```python
from build123d import *

# Parameters (mm, degrees)
F1_DEPTH = 76.2
F3_DEPTH = 38.101


with BuildPart() as f1:
    # F0 (on Front) → F1 (new body)
    with BuildSketch(Plane.XZ):
        Polygon((0, 101.6), (0, 0), (152.4, 0), (152.4, 38.1), (38.1, 38.1), (38.1, 101.6), align=None)
    extrude(amount=F1_DEPTH)

    # F2 (on face) → F3 (cut, through all)
    with BuildSketch(Plane.YZ.offset(38.1)):
        Polygon((-76.2, 69.85), (-38.1, 101.6), (-76.2, 101.6), align=None)
    extrude(amount=-F3_DEPTH, mode=Mode.SUBTRACT)


solid = f1.part
```
Here's how the part is built. I have some questions about the finished solid (model axes, mm). A direction names the side the tool comes from. Coordinates: 2 decimals unless noted, no trailing zeros. Write each loop counter-clockwise with the first axis right and the second up, starting at its lowest first coordinate (ties: lowest second). Pieces come first, ordered by that corner, then holes. Notation, with made-up numbers: (-5.5, 25.25) -> (16.5, 25.25) arc R17 cw to (16.5, 32.25) -> close; hole circle Ø2 at (-18.75, 16.5). An arc over 180 degrees is marked (long way). Use a Markdown table: item, result. Add a question column.
(1) If we section it at B-B, the plane x = 129.5: Write out the boundary of the cut face in (y, z).
(2) If we section it at A-A, the plane y = -55.5: Write out the boundary of the cut face in (x, z).
(3) I'm going to push flat-ended pins straight in: P1, Ø23, axis at x = 112, y = -30, coming from the +Z side; P2, Ø8, axis at y = -50, z = 51, coming from the +X side. Where does each tip first touch, or does it pass through?
(4) Please list where these lines run through material, in increasing order: line 1 (Z direction, x = 100, y = -9.5); line 2 (Y direction, x = 38, z = 95).
(5) If we section it at D-D, the plane y = -11: Write out the boundary of the cut face in (x, z).
(6) For faces 1 (the flat face through (38.1, -38, 69)), 2 (the flat face through (19, -19, 101.6)), which set-ups out of +Z, -Z, +X, -X, +Y, -Y let a thin tool reach every point of the face, with its end or its side?
(7) If we section it at C-C, the plane z = 79: Write out the boundary of the cut face in (x, y), and give its area (3 significant figures).
Outcome:
| question | item | result |
|---|---|---|
| 1 | outline | (-76.2, 0) -> (0, 0) -> (0, 38.1) -> (-76.2, 38.1) -> close |
| 2 | outline | (0, 0) -> (152.4, 0) -> (152.4, 38.1) -> (38.1, 38.1) -> (38.1, 87.1) -> (0, 87.1) -> close |
| 3 | P1 | stops at z = 38.1 |
| 3 | P2 | stops at x = 38.1 |
| 4 | line 1 | z = 0 to 38.1 |
| 4 | line 2 | y = -46.02 to 0 |
| 5 | outline | (0, 0) -> (152.4, 0) -> (152.4, 38.1) -> (38.1, 38.1) -> (38.1, 101.6) -> (0, 101.6) -> close |
| 6 | face 1 | +Z, +X, +Y, -Y |
| 6 | face 2 | +Z, +X, -X, +Y, -Y |
| 7 | outline | (0, -65.22) -> (38.1, -65.22) -> (38.1, 0) -> (0, 0) -> close |
| 7 | area | 2,480 mm^2 |
